from build123d import *

# Parameters (mm, degrees)
CYLINDER001_R     = 17.5
CYLINDER001_DEPTH = 12
FILLET001_R       = 5
BOX003_W          = 14
BOX003_H          = 17
BOX003_DEPTH      = 12
CYLINDER002_R     = 9.1
CYLINDER002_DEPTH = 12
FILLET002_R       = 5
BOX004_W          = 4
BOX004_H          = 19
BOX004_DEPTH      = 12
SKETCH006_R       = 3
HOLE_DEPTH        = 25


with BuildPart() as part:
    # Cylinder001 → Cylinder001 (join)
    with BuildSketch(Plane.XY):
        Circle(CYLINDER001_R)
    extrude(amount=CYLINDER001_DEPTH)

    # Fillet001
    fillet001_edges = [part.edges().sort_by_distance(p)[0] for p in [
        (-17.5, 0, 12),
    ]]
    fillet(fillet001_edges, radius=FILLET001_R)

    # Box003 → Box003 (join)
    with BuildSketch(Plane(origin=(-7, -27, 0), x_dir=(1, 0, 0), z_dir=(0, 0, 1))):
        with Locations((7, 8.5)):
            Rectangle(BOX003_W, BOX003_H)
    extrude(amount=BOX003_DEPTH)

    # Cylinder002 → Cylinder002 (cut)
    with BuildSketch(Plane.XY):
        Circle(CYLINDER002_R)
    extrude(amount=CYLINDER002_DEPTH, mode=Mode.SUBTRACT)

    # Fillet002
    fillet002_edges = [part.edges().sort_by_distance(p)[0] for p in [
        (0, -27, 12),
        (0, -27, 0),
    ]]
    fillet(fillet002_edges, radius=FILLET002_R)

    # Box004 → Box004 (cut)
    with BuildSketch(Plane(origin=(-2, -27, 0), x_dir=(1, 0, 0), z_dir=(0, 0, 1))):
        with Locations((2, 9.5)):
            Rectangle(BOX004_W, BOX004_H)
    extrude(amount=BOX004_DEPTH, mode=Mode.SUBTRACT)

    # Sketch006 (on Face1 of Box004) → Hole (cut)
    with BuildSketch(Plane(origin=(7, -27, 0), x_dir=(0, 1, 0), z_dir=(1, 0, 0))):
        with Locations((5.5, 6)):
            Circle(SKETCH006_R)
    extrude(amount=-HOLE_DEPTH, mode=Mode.SUBTRACT)


with BuildPart() as part_1:
    # Body004 placement: moved
    add(part.part.moved(Location((-265, 0, 75))))


solid = part_1.part
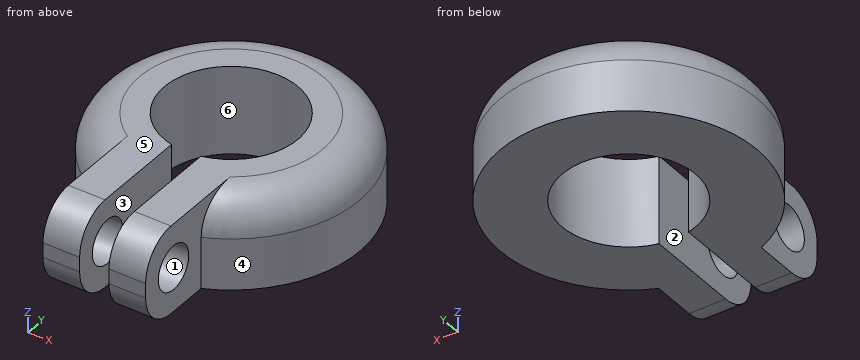
Here's how the part is built. I have some questions about the finished solid (model axes, mm). Face numbers are marked on the shaded views. A direction names the side the tool comes from. Round coordinates to 2 decimals unless told otherwise and drop trailing zeros. Order: outer loops, then holes, each group sorted by start corner. A loop starts at its lowest first (then second) coordinate and runs counter-clockwise, first axis right, second up. Notation, with made-up numbers: M 86.25,57.5 L 102.25,57.5 A21 cw 102.25,68.5 Z; hole C -31,6 d7. An arc over 180 degrees is marked long. One line per question, with ' | ' between items.
1) Imagine slicing it at B-B, the plane y = 0. Write out the boundary of the cut face in (x, z), plus the area to 3 significant figures.
Checked values:
outline: M -282.5,75 L -274.1,75 L -274.1,87 L -277.5,87 A5 ccw -282.5,82 Z; M -255.9,75 L -247.5,75 L -247.5,82 A5 ccw -252.5,87 L -255.9,87 Z | area: 191 mm²
2) We'd pull the mould along X, two halves only. Please class the marked faces 3, 4, 5 and 6: released by +X, released by -X, zero draft, split by the parting line, or undercut.
Checked values:
face 3: undercut | face 4: split by the parting line | face 5: zero draft | face 6: undercut
3) Imagine slicing it at D-D, the plane x = -258.5. Count the separate pieces of the cut face and the enclosed holes in it, plus the area to 3 significant figures.
Checked values:
separate pieces: 2 | enclosed holes: 1 | area: 321 mm²
4) On a 3-axis mill with a long thin cutter (end or side, diameter ignored), from which of +Z, -Z, +X, -X, +Y, -Y can I reach the whole of each face in a straight line? I mean the marked faces 1 and 2. Say none if no direction works.
Checked values:
face 1: +X, -X | face 2: +Z, -Z, -Y
5) Imagine slicing it at A-A, the plane z = 81. Write out the boundary of the cut face in (x, y), plus the area to 3 significant figures.
Checked values:
outline: M -272,-27 L -267,-27 L -267,-24.5 L -272,-24.5 Z; M -272,-18.5 L -267,-18.5 L -267,-8.88 A9.1 cw long -263,-8.88 L -263,-18.5 L -258,-18.5 L -258,-16.04 A17.5 ccw long -272,-16.04 Z; M -263,-27 L -258,-27 L -258,-24.5 L -263,-24.5 Z | area: 710 mm²
6) I need wall thicknesses on line 1 (Z direction, x = -261.8, y = -21.5); line 2 (X direction, y = -17, z = 82.25); line 3 (Y direction, x = -269, z = 82). Which ranges of each line are inside material? Lowest first, please.
Checked values:
line 1: z = 75 to 78, 84 to 87 | line 2: x = -272 to -267, -263 to -258 | line 3: y = -27 to -24.33, -18.67 to -8.17, 8.17 to 17.04
7) I'm going to push flat-ended pins straight in: pin 1 Ø4 at (y, z) = (7, 81.5) entering from -X; pin 2 Ø6 at (y, z) = (-20, 80) entering from -X; pin 3 Ø2 at (y, z) = (2.5, 85.5) entering from -X. Where does each tip first touch, or does it pass through?
Checked values:
pin 1: stops at x = -281.77 | pin 2: stops at x = -272 | pin 3: stops at x = -281.66
8) Imagine slicing it at C-C, the plane x = -265. Write out the boundary of the cut face in (y, z), plus the area to 3 significant figures.
Checked values:
outline: M 9.1,75 L 17.5,75 L 17.5,82 A5 ccw 12.5,87 L 9.1,87 Z | area: 95.4 mm²
